CAD build for the part. Positions are in the model's coordinates, mm. A direction names the side the tool comes from. Round coordinates to 2 decimals unless told otherwise and drop trailing zeros. Loops run counter-clockwise (first coordinate to the right, second up) from the corner with the lowest first, then second, coordinate; pieces in that order, holes last. Notation, with made-up numbers: (-0.75, 76.25) -> (4.25, 76.25) arc R27 ccw to (4.25, 115.25) -> close; hole circle Ø3 at (36.5, 58.5). An arc over 180 degrees is marked (long way). Answer as CSV lines item,"result".
```python
from build123d import *

# Parameters (mm, degrees)
SKETCH1_W                   = 25.4
SKETCH1_H                   = 50.8
BOSS_EXTRUDE1_DEPTH         = 76.2
F_1_4_0_25_DIAMETER_HOLE1_D = 6.35
F_10_32_TAPPED_HOLE1_D      = 4.0386
F_10_32_TAPPED_HOLE1_DEPTH  = 13.716
F_10_32_TAPPED_HOLE1_TIP    = 1.213317848
CUT_EXTRUDE1_DEPTH          = 85.242269675
SKETCH9_W                   = 19.05
SKETCH9_H                   = 44.45
CUT_EXTRUDE2_DEPTH          = 156.02325632


with BuildPart() as part:
    # Sketch1 → Boss-Extrude1 (new, symmetric)
    with BuildSketch(Plane.XY):
        Rectangle(SKETCH1_W, SKETCH1_H)
    extrude(amount=BOSS_EXTRUDE1_DEPTH, both=True)

    # 1/4 (0.25) Diameter Hole1 (through all)
    with Locations(Plane(origin=(12.7, 0, 0), x_dir=(0, 0, -1), z_dir=(1, 0, 0))):
        with Locations((-63.5, 17.4625), (16.002, 17.4625), (16.002, -17.5895), (-63.5, -17.5895)):
            Hole(F_1_4_0_25_DIAMETER_HOLE1_D / 2)

    # #10-32 Tapped Hole1
    with Locations(Plane(origin=(0, 25.4, 0), x_dir=(1, 0, 0), z_dir=(0, 1, 0))):
        with Locations((0, 63.5), (0, 50.8)):
            Hole(F_10_32_TAPPED_HOLE1_D / 2, depth=F_10_32_TAPPED_HOLE1_DEPTH)
            with Locations((0, 0, -(F_10_32_TAPPED_HOLE1_DEPTH + F_10_32_TAPPED_HOLE1_TIP / 2))):  # 118° drill point
                Cone(0, F_10_32_TAPPED_HOLE1_D / 2, F_10_32_TAPPED_HOLE1_TIP, mode=Mode.SUBTRACT)

    # Sketch8 → Cut-Extrude1 (cut, through all)
    with BuildSketch(Plane(origin=(12.7, 0, 0), x_dir=(0, 0, -1), z_dir=(1, 0, 0))):
        Polygon((76.2, 25.4), (71.12, -25.4), (76.2, -25.4), align=None)
    extrude(amount=-CUT_EXTRUDE1_DEPTH, mode=Mode.SUBTRACT)

    # Sketch9 → Cut-Extrude2 (cut, through all)
    with BuildSketch(Plane.XY.offset(76.2)):
        Rectangle(SKETCH9_W, SKETCH9_H)
    extrude(amount=-CUT_EXTRUDE2_DEPTH, mode=Mode.SUBTRACT)


solid = part.part
```
Q1. Tool access for faces 5 (the cylindrical face through (-11.13, 20.61, -16.42)), 6 (the cylindrical face through (0.263, 23.79, -65.502)), 7 (the flat face through (0, -22.225, 3)): list every direction of +Z, -Z, +X, -X, +Y, -Y with a clear straight run to the whole face (end or side of a thin tool).
Results:
face 5,"+X, -X"
face 6,"+Y"
face 7,"+Z, -Z"
Q2. Slice it at D-D, the plane z = 63.5. Give the cut face in (x, y) (1 decimal).
Results:
outline,"(-12.7, -25.4) -> (12.7, -25.4) -> (12.7, -20.8) -> (9.5, -20.8) -> (9.5, -22.2) -> (-9.5, -22.2) -> (-9.5, -20.8) -> (-12.7, -20.8) -> close; (-12.7, -14.4) -> (-9.5, -14.4) -> (-9.5, 14.3) -> (-12.7, 14.3) -> close; (-12.7, 20.6) -> (-9.5, 20.6) -> (-9.5, 22.2) -> (9.5, 22.2) -> (9.5, 20.6) -> (12.7, 20.6) -> (12.7, 25.4) -> (-12.7, 25.4) -> close; (9.5, -14.4) -> (12.7, -14.4) -> (12.7, 14.3) -> (9.5, 14.3) -> close"
Q3. Slice it at C-C, the plane x = -6.5. Give the cut face in (y, z) (1 decimal), and give its area (3 significant figures).
Results:
outline,"(-25.4, -71.1) -> (-22.2, -71.4) -> (-22.2, 76.2) -> (-25.4, 76.2) -> close; (22.2, -75.9) -> (25.4, -76.2) -> (25.4, 76.2) -> (22.2, 76.2) -> close"
area,"952 mm2"
Q4. Slice it at B-B, the plane y = -8.5. Give the cut face in (x, z) (3 decimals).
Results:
outline,"(-12.7, -72.81) -> (-9.525, -72.81) -> (-9.525, 76.2) -> (-12.7, 76.2) -> close; (9.525, -72.81) -> (12.7, -72.81) -> (12.7, 76.2) -> (9.525, 76.2) -> close"
Q5. Slice it at A-A, the plane x = 0. Give the cut face in (y, z) (1 decimal), and give its area (3 significant figures).
Results:
outline,"(-25.4, -71.1) -> (-22.2, -71.4) -> (-22.2, 76.2) -> (-25.4, 76.2) -> close; (22.2, -75.9) -> (25.4, -76.2) -> (25.4, -65.5) -> (22.2, -65.5) -> close; (22.2, -61.5) -> (25.4, -61.5) -> (25.4, -52.8) -> (22.2, -52.8) -> close; (22.2, -48.8) -> (25.4, -48.8) -> (25.4, 76.2) -> (22.2, 76.2) -> close"
area,"926 mm2"
Q6. Two-plate mould, pull along Y, no slides. Class faces 1 (the flat face through (12.7, 0, 1)), 2 (the flat face through (0, 22.225, 1)), 3 (the cylindrical face through (11.09, 20.61, -16.42)), 4 (the flat face through (0, -25.4, 4)): pulls with the +Y half, pulls with the -Y half, needs draft (parallel to the pull), parting line crosses it, or undercut.
Results:
face 1,"needs draft"
face 2,"undercut"
face 3,"undercut"
face 4,"pulls with the -Y half"
Q7. Probe L1, parallel to Y at x = 11.5, z = 63.5; L2, parallel to Y at x = -6.75, z = 6.5 (3 decimals); L3, parallel to X at y = 1, z = 53 (3 decimals). List the from-to ranges inside material, lowest first. Write a range as [from, to].
Results:
L1,"[-25.4, -20.76], [-14.41, 14.29], [20.64, 25.4]"
L2,"[-25.4, -22.225], [22.225, 25.4]"
L3,"[-12.7, -9.525], [9.525, 12.7]"
Q8. Drop flat-ended pins along their axis: pin 1 Ø10 at (x, y) = (8, 8.5) entering from -Z; pin 2 Ø3.5 at (x, z) = (0, -63.5) entering from +Y (3 decimals). Give the stop position or say it passes through.
Results:
pin 1,"z = -74.99"
pin 2,"y = -22.225"
